from build123d import *

# Parameters (mm, degrees)
SKETCH1_W           = 10
SKETCH1_H           = 10
BOSS_EXTRUDE1_DEPTH = 90
SKETCH2_R           = 2.5
BOSS_EXTRUDE2_DEPTH = 10
SKETCH3_R           = 2.5
CUT_EXTRUDE1_DEPTH  = 101.623058987


with BuildPart() as part:
    # Sketch1 → Boss-Extrude1 (new body)
    with BuildSketch(Plane(origin=(0, 0, 0), x_dir=(1, 0, 0), z_dir=(0, 1, 0))):
        Rectangle(SKETCH1_W, SKETCH1_H)
    extrude(amount=BOSS_EXTRUDE1_DEPTH)

    # Sketch2 → Boss-Extrude2 (add)
    with BuildSketch(Plane(origin=(0, 90, 0), x_dir=(1, 0, 0), z_dir=(0, 1, 0))):
        with Locations(Location((0, 0, 0), (0, 0, 270))):
            Circle(SKETCH2_R)
    extrude(amount=BOSS_EXTRUDE2_DEPTH)

    # Sketch3 → Cut-Extrude1 (cut, through all)
    with BuildSketch(Plane(origin=(5, 0, 0), x_dir=(0, 0, -1), z_dir=(1, 0, 0))):
        with Locations((0, 5)):
            Circle(SKETCH3_R)
    extrude(amount=-CUT_EXTRUDE1_DEPTH, mode=Mode.SUBTRACT)


solid = part.part
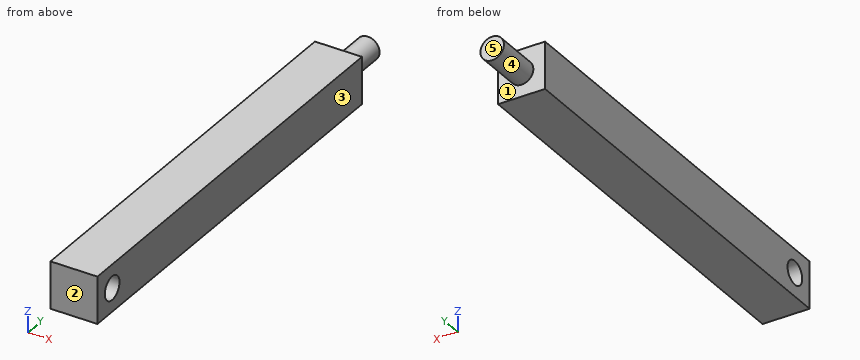
Verification items for the finished model (mm, model axes). Face numbers are marked on the shaded views. A direction names the side the tool comes from. Round coordinates to 2 decimals unless told otherwise and drop trailing zeros. Loops run counter-clockwise (first coordinate to the right, second up) from the corner with the lowest first, then second, coordinate; pieces in that order, holes last. Notation, with made-up numbers: (82, -18.75) - (124, -18.75) arc R33 ccw to (124, 17.25) - close; hole circle Ø4 at (61.5, 72). An arc over 180 degrees is marked (long way). Write item = value, one per line.
Q1. Mould release check, pull along X, two halves, no side actions. Record for the marked faces 3, 4 and 5: +X half, -X half, draft (parallel to the pull), parting line (faces both ways), or undercut.
Here are the results:
face_3 = +X half
face_4 = parting line
face_5 = draft
Q2. Sectioned sample at D-D on x = 4. Record the boundary of the cut face in (y, z).
Here are the results:
outline = (0, -5) - (90, -5) - (90, 5) - (0, 5) - close; hole circle Ø5 at (5, 0)
Q3. Material ranges on L1, parallel to Y at x = -0.5, z = 0; L2, parallel to Y at x = 0, z = 2; L3, parallel to Y at x = -4, z = -2.75, recorded low to high.
Here are the results:
L1 = 0 to 2.5, 7.5 to 100
L2 = 0 to 3.5, 6.5 to 100
L3 = 0 to 90
Q4. Tool access check on the marked faces 1 and 2. Record the directions out of +Z, -Z, +X, -X, +Y, -Y that give a thin tool (end or side, any length) a straight path to the whole face; none if there is none.
Here are the results:
face_1 = +Y
face_2 = +Z, -Z, +X, -X, -Y
Q5. Sectioned sample at C-C on x = 0. Record the boundary of the cut face in (y, z), plus the area to 3 significant figures.
Here are the results:
outline = (0, -5) - (90, -5) - (90, -2.5) - (100, -2.5) - (100, 2.5) - (90, 2.5) - (90, 5) - (0, 5) - close; hole circle Ø5 at (5, 0)
area = 930 mm^2
Q6. Depth check by flat-ended pin: pin 1 (4 mm diameter, centred on y = 5, z = 0, fed in from -X). Enter the tip coordinate at first touch or a pass-through.
Here are the results:
pin_1 = through
Q7. Sectioned sample at B-B on z = 0. Record the boundary of the cut face in (x, y).
Here are the results:
outline = (-5, 0) - (5, 0) - (5, 2.5) - (-5, 2.5) - close; (-5, 7.5) - (5, 7.5) - (5, 90) - (2.5, 90) - (2.5, 100) - (-2.5, 100) - (-2.5, 90) - (-5, 90) - close
Q8. Sectioned sample at A-A on y = 5. Record the boundary of the cut face in (x, z), plus the area to 3 significant figures.
Here are the results:
outline = (-5, -5) - (5, -5) - (5, -2.5) - (-5, -2.5) - close; (-5, 2.5) - (5, 2.5) - (5, 5) - (-5, 5) - close
area = 50.0 mm^2
